Drawing for the job (mm, zero at the part's lowest x, y, z). A direction names the side the tool comes from. Give positions to 0.01 mm unless a question says otherwise; leave off trailing zeros. Loops run counter-clockwise (first coordinate to the right, second up) from the corner with the lowest first, then second, coordinate; pieces in that order, holes last.
1) Two-plate mould, pull along X, no slides. Class the marked faces 1, 2, 3 and 4: +X half, -X half, draft (parallel to the pull), parting line (faces both ways), or undercut.
2) Band-saw the part on D-D on x = 3. List the corners of the cut face in (y, z).
3) Wall check: line 1 (X direction, y = 12.25, z = 0.6); line 2 (X direction, y = 15.75, z = 2.75); line 3 (Y direction, x = 3, z = 2.35). Give the ranges that are in metal, low to high.
4) Band-saw the part on C-C on z = 1.6. State how many separate pieces and enclosed holes the cut face has, then the cut area to 3 significant figures.
5) Band-saw the part on B-B on y = 12.25. List the corners of the cut face in (x, z), then the cut area to 3 significant figures.
6) Band-saw the part on A-A on x = 14. List the corners of the cut face in (y, z), then the cut area to 3 significant figures.
7) Flat gauge pins, fed straight in: P1, Ø0.9, axis at x = 39, z = 2, coming from the +Y side; P2, Ø6, axis at x = 14.5, y = 9.5, coming from the -Z side; P3, Ø0.9, axis at y = 2, z = 1.5, coming from the +X side; P4, Ø0.9, axis at x = 34.5, z = 1.5, coming from the -Y side. Where does each tip first touch, or does it go through?
8) 3-axis set-ups, long thin cutter, end or side, ignore diameter. For the marked faces 5, 6, 7 and 8: which of +Z, -Z, +X, -X, +Y, -Y reach the whole face in a straight line?
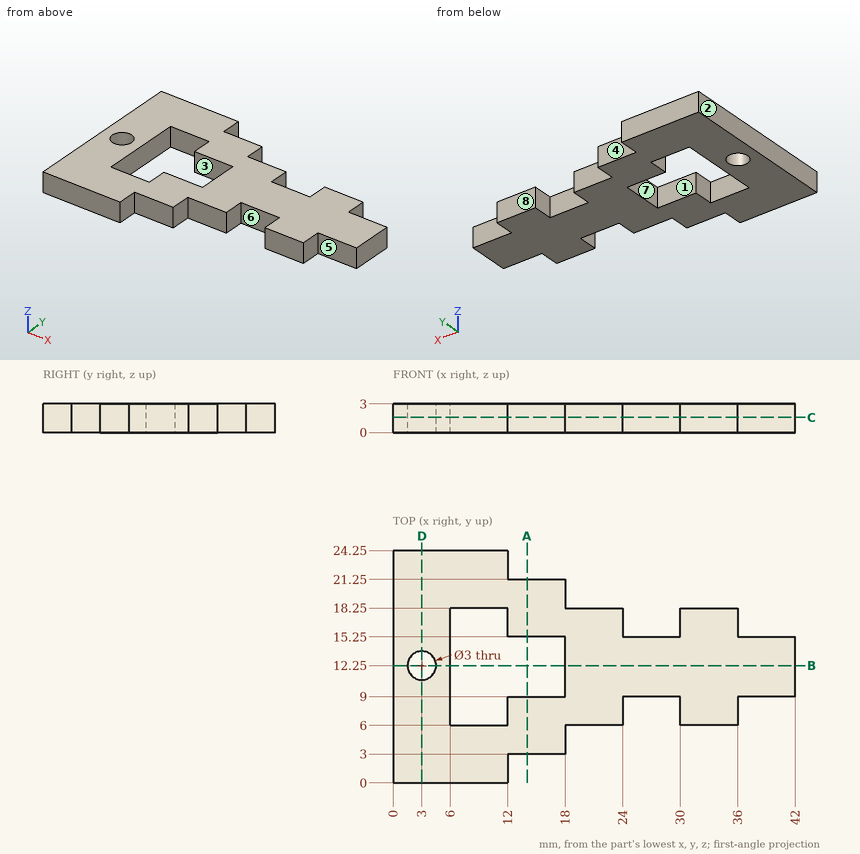
Findings below:
1. face 1: undercut
1. face 2: -X half
1. face 3: undercut
1. face 4: draft
2. outline: (0, 0) - (10.75, 0) - (10.75, 3) - (0, 3) - close; (13.75, 0) - (24.25, 0) - (24.25, 3) - (13.75, 3) - close
3. line 1: x = 0 to 1.5, 4.5 to 6, 18 to 42
3. line 2: x = 0 to 6, 12 to 24, 30 to 36
3. line 3: y = 0 to 10.75, 13.75 to 24.25
4. separate pieces: 1
4. enclosed holes: 2
4. area: 504 mm2
5. outline: (0, 0) - (1.5, 0) - (1.5, 3) - (0, 3) - close; (4.5, 0) - (6, 0) - (6, 3) - (4.5, 3) - close; (18, 0) - (42, 0) - (42, 3) - (18, 3) - close
5. area: 81.0 mm2
6. outline: (3, 0) - (9, 0) - (9, 3) - (3, 3) - close; (15.25, 0) - (21.25, 0) - (21.25, 3) - (15.25, 3) - close
6. area: 36.0 mm2
7. P1: stops at y = 15.25
7. P2: stops at z = 0
7. P3: stops at x = 12
7. P4: stops at y = 6
8. face 5: +Z, -Z, +X, -Y
8. face 6: +Z, -Z, -Y
8. face 7: +Z, -Z
8. face 8: +Z, -Z, +X, +Y
